from build123d import *

# Parameters (mm, degrees)
SKETCH1_W                    = 544
SKETCH1_H                    = 185
BASE_FLANGE1_DEPTH           = 3
EDGE_FLANGE1_STRIP_W         = 22
EDGE_FLANGE1_STRIP_H         = 3
EDGE_FLANGE1_STRIP_CUT_DEPTH = 544
EDGE_FLANGE1_DEPTH           = 544
EDGE_FLANGE2_STRIP_W         = 22
EDGE_FLANGE2_STRIP_H         = 3
EDGE_FLANGE2_STRIP_CUT_DEPTH = 544
EDGE_FLANGE2_DEPTH           = 544
EDGE_FLANGE3_STRIP_W         = 22
EDGE_FLANGE3_STRIP_H         = 3
EDGE_FLANGE3_STRIP_CUT_DEPTH = 544
EDGE_FLANGE3_DEPTH           = 544
EDGE_FLANGE4_STRIP_W         = 22
EDGE_FLANGE4_STRIP_H         = 3
EDGE_FLANGE4_STRIP_CUT_DEPTH = 544
EDGE_FLANGE4_DEPTH           = 544
EDGE_FLANGE5_STRIP_W         = 22
EDGE_FLANGE5_STRIP_H         = 3
EDGE_FLANGE5_STRIP_CUT_DEPTH = 169
EDGE_FLANGE5_DEPTH           = 169
EDGE_FLANGE6_STRIP_W         = 22
EDGE_FLANGE6_STRIP_H         = 3
EDGE_FLANGE6_STRIP_CUT_DEPTH = 169
EDGE_FLANGE6_DEPTH           = 169
SKETCH26_R                   = 4.25
CUT_EXTRUDE1_DEPTH           = 10
SKETCH27_R                   = 4.25
CUT_EXTRUDE2_DEPTH           = 10


# Sheet-metal steps are written as plain solids
with BuildPart() as part:
    # Sketch1 → Base-Flange1 (new body)
    with BuildSketch(Plane.XY):
        with Locations((-108.962758621, -57.524490421)):
            Rectangle(SKETCH1_W, SKETCH1_H)
        with BuildLine():
            Line((152.537241379, 4.975509579), (122.537241379, 4.975509579))
            ThreePointArc((122.537241379, 4.975509579), (117.537241379, 9.975509579), (122.537241379, 14.975509579))
            Line((122.537241379, 14.975509579), (152.537241379, 14.975509579))
            ThreePointArc((152.537241379, 14.975509579), (157.537241379, 9.975509579), (152.537241379, 4.975509579))
        make_face(mode=Mode.SUBTRACT)
        with BuildLine():
            Line((57.537241379, 4.975509579), (27.537241379, 4.975509579))
            ThreePointArc((27.537241379, 4.975509579), (22.537241379, 9.975509579), (27.537241379, 14.975509579))
            Line((27.537241379, 14.975509579), (57.537241379, 14.975509579))
            ThreePointArc((57.537241379, 14.975509579), (62.537241379, 9.975509579), (57.537241379, 4.975509579))
        make_face(mode=Mode.SUBTRACT)
        with BuildLine():
            Line((152.537241379, -80.024490421), (122.537241379, -80.024490421))
            ThreePointArc((122.537241379, -80.024490421), (117.537241379, -75.024490421), (122.537241379, -70.024490421))
            Line((122.537241379, -70.024490421), (152.537241379, -70.024490421))
            ThreePointArc((152.537241379, -70.024490421), (157.537241379, -75.024490421), (152.537241379, -80.024490421))
        make_face(mode=Mode.SUBTRACT)
        with BuildLine():
            Line((57.537241379, -80.024490421), (27.537241379, -80.024490421))
            ThreePointArc((27.537241379, -80.024490421), (22.537241379, -75.024490421), (27.537241379, -70.024490421))
            Line((27.537241379, -70.024490421), (57.537241379, -70.024490421))
            ThreePointArc((57.537241379, -70.024490421), (62.537241379, -75.024490421), (57.537241379, -80.024490421))
        make_face(mode=Mode.SUBTRACT)
    extrude(amount=-BASE_FLANGE1_DEPTH)

    # Edge-Flange1 strip (across the edge) → Edge-Flange1 strip cut (cut)
    with BuildSketch(Plane(origin=(-380.962758621, 34.975509579, -3), x_dir=(0, -1, 0), z_dir=(1, 0, 0))):
        with Locations((-3, -1.5)):
            Rectangle(EDGE_FLANGE1_STRIP_W, EDGE_FLANGE1_STRIP_H)
    extrude(amount=EDGE_FLANGE1_STRIP_CUT_DEPTH, mode=Mode.SUBTRACT)

    # Edge-Flange1 section (across the edge) → Edge-Flange1 (add)
    with BuildSketch(Plane(origin=(-380.962758621, 34.975509579, -3), x_dir=(0, -1, 0), z_dir=(1, 0, 0))):
        with BuildLine():
            Line((0, 5), (0, 22))
            Line((0, 22), (3, 22))
            Line((3, 22), (3, 5))
            ThreePointArc((3, 5), (4.464466094, 1.464466094), (8, 0))
            Line((8, 0), (8, -3))
            ThreePointArc((8, -3), (2.343145751, -0.656854249), (0, 5))
        make_face()
    extrude(amount=EDGE_FLANGE1_DEPTH)

    # Edge-Flange2 strip (across the edge) → Edge-Flange2 strip cut (cut)
    with BuildSketch(Plane(origin=(163.037241379, -150.024490421, -3), x_dir=(0, 1, 0), z_dir=(-1, 0, 0))):
        with Locations((-3, -1.5)):
            Rectangle(EDGE_FLANGE2_STRIP_W, EDGE_FLANGE2_STRIP_H)
    extrude(amount=EDGE_FLANGE2_STRIP_CUT_DEPTH, mode=Mode.SUBTRACT)

    # Edge-Flange2 section (across the edge) → Edge-Flange2 (add)
    with BuildSketch(Plane(origin=(163.037241379, -150.024490421, -3), x_dir=(0, 1, 0), z_dir=(-1, 0, 0))):
        with BuildLine():
            Line((0, 5), (0, 22))
            Line((0, 22), (3, 22))
            Line((3, 22), (3, 5))
            ThreePointArc((3, 5), (4.464466094, 1.464466094), (8, 0))
            Line((8, 0), (8, -3))
            ThreePointArc((8, -3), (2.343145751, -0.656854249), (0, 5))
        make_face()
    extrude(amount=EDGE_FLANGE2_DEPTH)

    # Edge-Flange3 strip (across the edge) → Edge-Flange3 strip cut (cut)
    with BuildSketch(Plane(origin=(-380.962758621, -150.024490421, -25), x_dir=(0, 0, 1), z_dir=(1, 0, 0))):
        with Locations((-3, -1.5)):
            Rectangle(EDGE_FLANGE3_STRIP_W, EDGE_FLANGE3_STRIP_H)
    extrude(amount=EDGE_FLANGE3_STRIP_CUT_DEPTH, mode=Mode.SUBTRACT)

    # Edge-Flange3 section (across the edge) → Edge-Flange3 (add)
    with BuildSketch(Plane(origin=(-380.962758621, -150.024490421, -25), x_dir=(0, 0, 1), z_dir=(1, 0, 0))):
        with BuildLine():
            Line((0, 5), (0, 27))
            Line((0, 27), (3, 27))
            Line((3, 27), (3, 5))
            ThreePointArc((3, 5), (4.464466094, 1.464466094), (8, 0))
            Line((8, 0), (8, -3))
            ThreePointArc((8, -3), (2.343145751, -0.656854249), (0, 5))
        make_face()
    extrude(amount=EDGE_FLANGE3_DEPTH)

    # Edge-Flange4 strip (across the edge) → Edge-Flange4 strip cut (cut)
    with BuildSketch(Plane(origin=(163.037241379, 34.975509579, -25), x_dir=(0, 0, 1), z_dir=(-1, 0, 0))):
        with Locations((-3, -1.5)):
            Rectangle(EDGE_FLANGE4_STRIP_W, EDGE_FLANGE4_STRIP_H)
    extrude(amount=EDGE_FLANGE4_STRIP_CUT_DEPTH, mode=Mode.SUBTRACT)

    # Edge-Flange4 section (across the edge) → Edge-Flange4 (add)
    with BuildSketch(Plane(origin=(163.037241379, 34.975509579, -25), x_dir=(0, 0, 1), z_dir=(-1, 0, 0))):
        with BuildLine():
            Line((0, 5), (0, 27))
            Line((0, 27), (3, 27))
            Line((3, 27), (3, 5))
            ThreePointArc((3, 5), (4.464466094, 1.464466094), (8, 0))
            Line((8, 0), (8, -3))
            ThreePointArc((8, -3), (2.343145751, -0.656854249), (0, 5))
        make_face()
    extrude(amount=EDGE_FLANGE4_DEPTH)

    # Edge-Flange5 strip (across the edge) → Edge-Flange5 strip cut (cut)
    with BuildSketch(Plane(origin=(163.037241379, 26.975509579, -3), x_dir=(-1, 0, 0), z_dir=(0, -1, 0))):
        with Locations((-6, -1.5)):
            Rectangle(EDGE_FLANGE5_STRIP_W, EDGE_FLANGE5_STRIP_H)
    extrude(amount=EDGE_FLANGE5_STRIP_CUT_DEPTH, mode=Mode.SUBTRACT)

    # Edge-Flange5 section (across the edge) → Edge-Flange5 (add)
    with BuildSketch(Plane(origin=(163.037241379, 26.975509579, -3), x_dir=(-1, 0, 0), z_dir=(0, -1, 0))):
        with BuildLine():
            Line((-3, 5), (-3, 22))
            Line((-3, 22), (0, 22))
            Line((0, 22), (0, 5))
            ThreePointArc((0, 5), (1.464466094, 1.464466094), (5, 0))
            Line((5, 0), (5, -3))
            ThreePointArc((5, -3), (-0.656854249, -0.656854249), (-3, 5))
        make_face()
    extrude(amount=EDGE_FLANGE5_DEPTH)

    # Edge-Flange6 strip (across the edge) → Edge-Flange6 strip cut (cut)
    with BuildSketch(Plane(origin=(-380.962758621, -142.024490421, -3), x_dir=(1, 0, 0), z_dir=(0, 1, 0))):
        with Locations((-6, -1.5)):
            Rectangle(EDGE_FLANGE6_STRIP_W, EDGE_FLANGE6_STRIP_H)
    extrude(amount=EDGE_FLANGE6_STRIP_CUT_DEPTH, mode=Mode.SUBTRACT)

    # Edge-Flange6 section (across the edge) → Edge-Flange6 (add)
    with BuildSketch(Plane(origin=(-380.962758621, -142.024490421, -3), x_dir=(1, 0, 0), z_dir=(0, 1, 0))):
        with BuildLine():
            Line((-3, 5), (-3, 22))
            Line((-3, 22), (0, 22))
            Line((0, 22), (0, 5))
            ThreePointArc((0, 5), (1.464466094, 1.464466094), (5, 0))
            Line((5, 0), (5, -3))
            ThreePointArc((5, -3), (-0.656854249, -0.656854249), (-3, 5))
        make_face()
    extrude(amount=EDGE_FLANGE6_DEPTH)

    # Sketch26 → Cut-Extrude1 (cut)
    with BuildSketch(Plane.XY.offset(-22)):
        with Locations((143.037241379, -165.524490421)):
            Circle(SKETCH26_R)
        with Locations((-360.962758621, -165.524490421)):
            Circle(SKETCH26_R)
    extrude(amount=-CUT_EXTRUDE1_DEPTH, mode=Mode.SUBTRACT)

    # Sketch27 → Cut-Extrude2 (cut)
    with BuildSketch(Plane.XY.offset(-22)):
        with Locations((143.037241379, 46.475509579)):
            Circle(SKETCH27_R)
        with Locations((-360.962758621, 46.475509579)):
            Circle(SKETCH27_R)
    extrude(amount=-CUT_EXTRUDE2_DEPTH, mode=Mode.SUBTRACT)


solid = part.part
Verification items for the finished model (mm, model axes). A direction names the side the tool comes from. Round coordinates to 2 decimals unless told otherwise and drop trailing zeros. Order: outer loops, then holes, each group sorted by start corner. A loop starts at its lowest first (then second) coordinate and runs counter-clockwise, first axis right, second up.
1. Release check for a two-part mould opening along X. For faces 5 (the flat face through (163.037, -153, -22)), 6 (the flat face through (-113, -56, -3)), 7 (the flat face through (-113, -56, 0)) record: +X half, -X half, draft (parallel to the pull), parting line (faces both ways), or undercut.
Final values:
face 5: +X half
face 6: undercut
face 7: draft
2. Section check B-B on x = -91. Record the cut outline in (y, z), then the cut area to 3 significant figures.
Final values:
outline: (-177.02, -25) - (-155.02, -25) arc R8 ccw to (-147.02, -17) - (-147.02, -8) arc R5 cw to (-142.02, -3) - (26.98, -3) arc R5 cw to (31.98, -8) - (31.98, -17) arc R8 ccw to (39.98, -25) - (61.98, -25) - (61.98, -22) - (39.98, -22) arc R5 cw to (34.98, -17) - (34.98, -8) arc R8 ccw to (26.98, 0) - (-142.02, 0) arc R8 ccw to (-150.02, -8) - (-150.02, -17) arc R5 cw to (-155.02, -22) - (-177.02, -22) - close
area: 816 mm2
3. Access from +Z, -Z, +X, -X, +Y, -Y to the whole of each face (thin tool, end or side, straight path). Record for faces 1 (the flat face through (163.037, -56, -17)), 2 (the flat face through (-380.963, 38, -22)), 3 (the flat face through (-105, 51, -22)), 4 (the flat face through (-113, -166, -22)).
Final values:
face 1: -Z
face 2: +Z, -Z, -X, +Y
face 3: +Z, +X, -X, +Y
face 4: +Z, +X, -X, -Y
4. Thickness scan on L1, parallel to Y at x = 8.5, z = -11.5; L2, parallel to X at y = -127.5, z = -11.75; L3, parallel to Z at x = 113, y = -66. Record the ranges inside material, lowest first.
Final values:
L1: y = -150.02 to -147.02, 31.98 to 34.98
L2: x = -383.96 to -380.96, 163.04 to 166.04
L3: z = -3 to 0
5. Go/stop test with flat-tipped pins: P1, Ø6, axis at x = -154, z = -5.5, coming from the +Y side; P2, Ø2.5, axis at x = 43, z = -1, coming from the +Y side; P3, Ø0.9, axis at x = -379, z = -1, coming from the +Y side. Record where each tip stops, or that it passes through.
Final values:
P1: stops at y = 34.98
P2: stops at y = 32.54
P3: stops at y = 31.57
6. Section check A-A on y = -135.5. Record the cut outline in (x, z), then the cut area to 3 significant figures.
Final values:
outline: (-383.96, -25) - (-380.96, -25) - (-380.96, -8) arc R5 cw to (-375.96, -3) - (158.04, -3) arc R5 cw to (163.04, -8) - (163.04, -25) - (166.04, -25) - (166.04, -8) arc R8 ccw to (158.04, 0) - (-375.96, 0) arc R8 ccw to (-383.96, -8) - close
area: 1,770 mm2
